Build history of the part. All positions in model axes, mm. A direction names the side the tool comes from. Round coordinates to 2 decimals unless told otherwise and drop trailing zeros. Loops run counter-clockwise (first coordinate to the right, second up) from the corner with the lowest first, then second, coordinate; pieces in that order, holes last. Notation, with made-up numbers: (-17.5, 11.5) - (39.5, 11.5) arc R10 ccw to (39.5, 28.5) - close; hole circle Ø4 at (57.5, 63). An arc over 180 degrees is marked (long way). One line per question, with ' | ' between items. Start each with the question number.
from build123d import *

# Parameters (mm, degrees)
SKETCH043_W     = 37.4
SKETCH043_H     = 41.56
PAD028_DEPTH    = 4
SKETCH044_W     = 34.2
SKETCH044_H     = 38.36
PAD029_DEPTH    = 2
SKETCH045_W     = 32.2
SKETCH045_H     = 36.36
POCKET024_DEPTH = 5
SKETCH046_W     = 34.2
SKETCH046_H     = 0.8
PAD030_DEPTH    = 0.8


with BuildPart() as part:
    # Sketch043 (on DatumPlane) → Pad028 (new body)
    with BuildSketch(Plane.XY.offset(6.7)):
        with Locations((16.9, 22.98)):
            Rectangle(SKETCH043_W, SKETCH043_H)
    extrude(amount=PAD028_DEPTH)

    # Sketch044 (on Face5 of Pad028) → Pad029 (join)
    with BuildSketch(Plane(origin=(0, 0, 6.7), x_dir=(1, 0, 0), z_dir=(0, 0, -1))):
        with Locations((16.9, -22.98)):
            Rectangle(SKETCH044_W, SKETCH044_H)
    extrude(amount=PAD029_DEPTH)

    # Sketch045 (on Face11 of Pad029) → Pocket024 (cut)
    with BuildSketch(Plane(origin=(0, 0, 4.7), x_dir=(1, 0, 0), z_dir=(0, 0, -1))):
        with Locations((16.9, -22.98)):
            Rectangle(SKETCH045_W, SKETCH045_H)
    extrude(amount=-POCKET024_DEPTH, mode=Mode.SUBTRACT)

    # Sketch046 (on Face9 of Pocket024) → Pad030 (join)
    with BuildSketch(Plane(origin=(0, 42.16, 6.7), x_dir=(-1, 0, 0), z_dir=(0, 1, 0))):
        with Locations((-16.9, -1.6)):
            Rectangle(SKETCH046_W, SKETCH046_H)
    extrude(amount=PAD030_DEPTH)


solid = part.part
1) Saw through at D-D on x = 33.5. Write the cut outline in (y, z).
2) Two-plate mould, pull along Y, no slides. Class faces 1 (the flat face through (17, 23, 10.7)), 2 (the flat face through (17, 43.76, 9)), 3 (the flat face through (17, 41.16, 7)): +Y half, -Y half, draft (parallel to the pull), parting line (faces both ways), or undercut.
3) Wall check: line 1 (X direction, y = 8.5, z = 6.35); line 2 (Y direction, x = 15, z = 9.3); line 3 (Y direction, x = 23.5, z = 5.3). Give the ranges that are in metal, low to high. Write a range as [from, to].
4) Tool access for faces 4 (the flat face through (-0.2, 23, 6)), 5 (the flat face through (34, 23, 6)), 6 (the flat face through (17, 4.8, 7)), 7 (the flat face through (17, 3.8, 6)), 8 (the flat face through (17, 42.16, 6)): list every direction of +Z, -Z, +X, -X, +Y, -Y with a clear straight run to the whole face (end or side of a thin tool).
5) Drop flat-ended pins along their axis: pin 1 (0.9 mm diameter, centred on x = 25.5, z = 5, fed in from +Y); pin 2 (0.6 mm diameter, centred on y = 18.5, z = 6, fed in from +X); pin 3 (1.5 mm diameter, centred on y = 22.5, z = 5.5, fed in from -X). Give the stop position or say it passes through.
6) Saw through at A-A on x = 16. Write the cut outline in (y, z), and give its area (3 significant figures).
7) Saw through at B-B on z = 7.55. Write the cut outline in (x, y), and give its area (3 significant figures).
8) Saw through at C-C on y = 40. Write the cut outline in (x, z).
Answer key:
1) outline: (2.2, 6.7) - (3.8, 6.7) - (3.8, 4.7) - (42.96, 4.7) - (42.96, 5.5) - (42.16, 5.5) - (42.16, 6.7) - (43.76, 6.7) - (43.76, 10.7) - (2.2, 10.7) - close
2) face 1: draft | face 2: +Y half | face 3: undercut
3) line 1: [-0.2, 0.8], [33, 34] | line 2: [2.2, 4.8], [41.16, 43.76] | line 3: [3.8, 4.8], [41.16, 42.96]
4) face 4: -Z, -X, +Y, -Y | face 5: -Z, +X, +Y, -Y | face 6: -Z | face 7: -Z, +X, -X, -Y | face 8: +X, -X, +Y
5) pin 1: y = 42.96 | pin 2: x = 34 | pin 3: x = -0.2
6) outline: (2.2, 6.7) - (3.8, 6.7) - (3.8, 4.7) - (4.8, 4.7) - (4.8, 9.7) - (41.16, 9.7) - (41.16, 4.7) - (42.96, 4.7) - (42.96, 5.5) - (42.16, 5.5) - (42.16, 6.7) - (43.76, 6.7) - (43.76, 10.7) - (2.2, 10.7) - close | area: 61.8 mm²
7) outline: (-1.8, 2.2) - (35.6, 2.2) - (35.6, 43.76) - (-1.8, 43.76) - close; hole (0.8, 4.8) - (33, 4.8) - (33, 41.16) - (0.8, 41.16) - close | area: 384 mm²
8) outline: (-1.8, 6.7) - (-0.2, 6.7) - (-0.2, 4.7) - (0.8, 4.7) - (0.8, 9.7) - (33, 9.7) - (33, 4.7) - (34, 4.7) - (34, 6.7) - (35.6, 6.7) - (35.6, 10.7) - (-1.8, 10.7) - close
